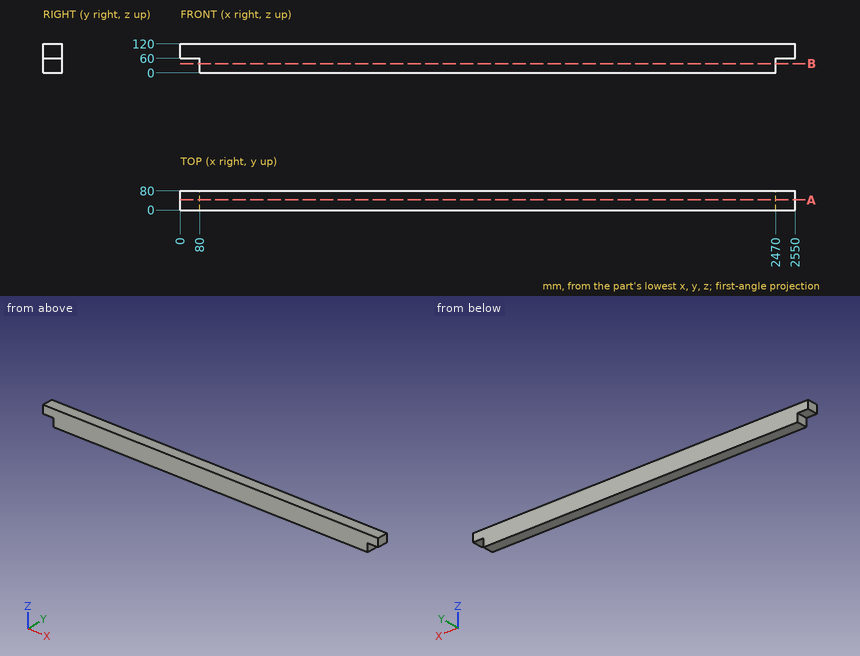
Study the drawing (mm; zero at the part's minimum x, y, z) and answer. Give positions to 0.01 mm unless a question says otherwise; leave off trailing zeros. Loops run counter-clockwise (first coordinate to the right, second up) from the corner with the lowest first, then second, coordinate; pieces in that order, holes last. Notation, with made-up numbers: M 88,-35.75 L 115,-35.75 A20 ccw 115,-11.75 Z; hole C 0,58 d1. An arc over 180 degrees is marked long. One line per item, written item: value. Start each with the question number.
1. Find section B-B (z = 39). Give the vertices of the cut face in (x, y).
2. Find the intervals of material crossed by probe 1 along X at (y, z) = (72.5, 59.5), in increasing order.
3. Each of these flat-tipped pins is pushed along its axis until it touches: P1, Ø24, axis at x = 2499.5, y = 20, coming from the -Z side; P2, Ø2, axis at y = 46.5, z = 21, coming from the +X side; P3, Ø2, axis at y = 31, z = 45.5, coming from the -X side. Where does it stop, or does it pass through?
4. Find section A-A (y = 43). Give the vertices of the cut face in (x, z), and give its area (3 significant figures).
Reported:
1. outline: M 80,0 L 2470,0 L 2470,80 L 80,80 Z
2. probe 1: x = 80 to 2470
3. P1: stops at z = 60
3. P2: stops at x = 2470
3. P3: stops at x = 80
4. outline: M 0,60 L 80,60 L 80,0 L 2470,0 L 2470,60 L 2550,60 L 2550,120 L 0,120 Z
4. area: 296,000 mm²
